The drawing under review shows one solid part. Ordinate dimensions are in mm from its lowest x, y, z. Give positions to 0.01 mm unless a question says otherwise; leave off trailing zeros. Loops run counter-clockwise (first coordinate to the right, second up) from the corner with the lowest first, then second, coordinate; pieces in that order, holes last. Notation, with made-up numbers: M 9,-37.5 L 55,-37.5 A29 cw 55,-6.5 Z; hole C 48.25,11.25 d5. An arc over 180 degrees is marked long. Answer as CSV lines item,"result".
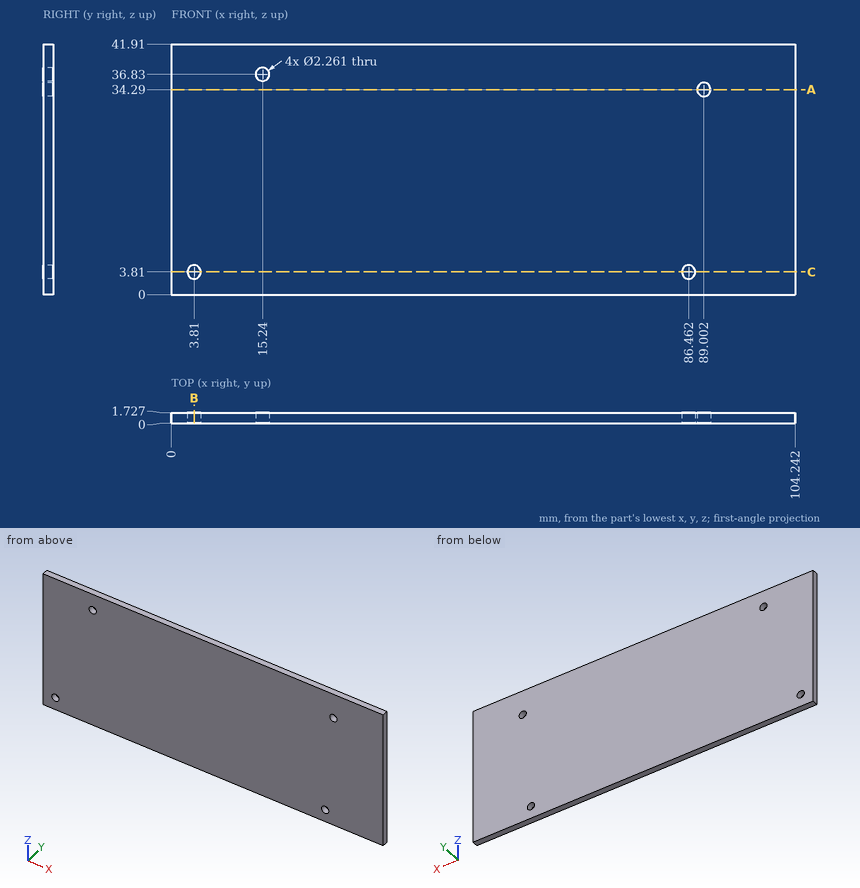
1. We need section A-A, the plane z = 34.29. Write out the cut boundary in (x, y), plus the area to 3 significant figures.
Answer block:
outline,"M 0,0 L 87.87,0 L 87.87,1.73 L 0,1.73 Z; M 90.13,0 L 104.24,0 L 104.24,1.73 L 90.13,1.73 Z"
area,"176 mm²"
2. We need section C-C, the plane z = 3.81. Write out the cut boundary in (x, y), plus the area to 3 significant figures.
Answer block:
outline,"M 0,0 L 2.68,0 L 2.68,1.73 L 0,1.73 Z; M 4.94,0 L 85.33,0 L 85.33,1.73 L 4.94,1.73 Z; M 87.59,0 L 104.24,0 L 104.24,1.73 L 87.59,1.73 Z"
area,"172 mm²"
3. We need section B-B, the plane x = 3.81. Write out the cut boundary in (y, z).
Answer block:
outline,"M 0,0 L 1.73,0 L 1.73,2.68 L 0,2.68 Z; M 0,4.94 L 1.73,4.94 L 1.73,41.91 L 0,41.91 Z"
4. To check wall thickness, follow L1, parallel to X at y = 0.4, z = 3.81; L2, parallel to Z at x = 3.81, y = 1.2; L3, parallel to X at y = 0.75, z = 36.83. State the ranges of each line that lie inside material, in increasing order. Write a range as [from, to].
Answer block:
L1,"[0, 2.68], [4.94, 85.33], [87.59, 104.24]"
L2,"[0, 2.68], [4.94, 41.91]"
L3,"[0, 14.11], [16.37, 104.24]"
